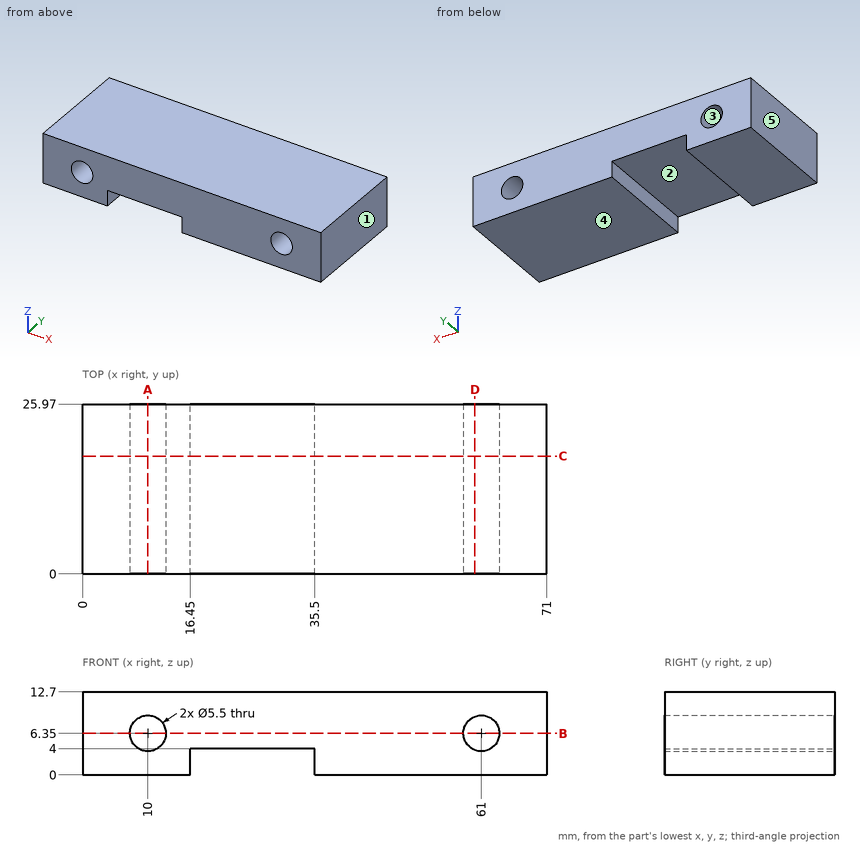
The drawing under review shows one solid part. Ordinate dimensions are in mm from its lowest x, y, z. A direction names the side the tool comes from. Give positions to 0.01 mm unless a question says otherwise; leave off trailing zeros. Loops run counter-clockwise (first coordinate to the right, second up) from the corner with the lowest first, then second, coordinate; pieces in that order, holes last. Notation, with made-up numbers: M 14,8 L 60,8 A22 cw 60,35 Z; hole C -15,16.25 d9. An arc over 180 degrees is marked long. One line per item, written item: value. Start each with the question number.
Q1. Machinability: for the marked faces 1 and 2, which of the approach directions +Z, -Z, +X, -X, +Y, -Y give a long, thin tool a straight path to every point of the face, cutting with its end or side? Answer none if there is none.
Q2. Add section B-B (z = 6.35). Give the boundary of the cut face in (x, y), and give its area (3 significant figures).
Q3. For L1, parallel to X at y = 2.5, z = 6.25; L2, parallel to X at y = 24.5, z = 4.5; L3, parallel to X at y = 10.75, z = 3, list the stretches that pass through material, from the lowest coordinate up.
Q4. Draft analysis for pull direction Z (two halves, no side actions). For the marked faces 3, 4 and 5, state which applies: released by +Z, released by -Z, zero draft, split by the parting line, or undercut.
Q5. Clearance check with a flat-ended pin moving along its axis: pin 1 Ø1.5 at (x, y) = (24.5, 15.5) entering from -Z. State where the tip first meets the part, or that it passes through.
Q6. Add section C-C (y = 18). Give the boundary of the cut face in (x, z).
Q7. Add section D-D (x = 60). Give the boundary of the cut face in (y, z).
Q8. Add section A-A (x = 10). Give the boundary of the cut face in (y, z), and give its area (3 significant figures).
Reply:
1. face 1: +Z, -Z, +X, +Y, -Y
1. face 2: -Z, +Y, -Y
2. outline: M 0,0 L 7.25,0 L 7.25,25.97 L 0,25.97 Z; M 12.75,0 L 58.25,0 L 58.25,25.97 L 12.75,25.97 Z; M 63.75,0 L 71,0 L 71,25.97 L 63.75,25.97 Z
2. area: 1,560 mm²
3. L1: 0 to 7.25, 12.75 to 58.25, 63.75 to 71
3. L2: 0 to 7.97, 12.03 to 58.97, 63.03 to 71
3. L3: 0 to 16.45, 35.5 to 71
4. face 3: undercut
4. face 4: released by -Z
4. face 5: zero draft
5. pin 1: z = 4
6. outline: M 0,0 L 16.45,0 L 16.45,4 L 35.5,4 L 35.5,0 L 71,0 L 71,12.7 L 0,12.7 Z; hole C 10,6.35 d5.5; hole C 61,6.35 d5.5
7. outline: M 0,0 L 25.97,0 L 25.97,3.79 L 0,3.79 Z; M 0,8.91 L 25.97,8.91 L 25.97,12.7 L 0,12.7 Z
8. outline: M 0,0 L 25.97,0 L 25.97,3.6 L 0,3.6 Z; M 0,9.1 L 25.97,9.1 L 25.97,12.7 L 0,12.7 Z
8. area: 187 mm²
